```python
from build123d import *

# Parameters (mm, degrees)
F0_W     = 101.6
F0_H     = 50.8
F1_DEPTH = 25.4
F2_W     = 50.8
F2_H     = 25.4
F3_DEPTH = 25.401


with BuildPart() as f1:
    # F0 (on Front) → F1 (new body)
    with BuildSketch(Plane.XZ):
        Rectangle(F0_W, F0_H)
    extrude(amount=F1_DEPTH)

    # F2 (on Front) → F3 (cut, through all)
    with BuildSketch(Plane.XZ):
        with Locations((25.4, 0)):
            Rectangle(F2_W, F2_H)
    extrude(amount=F3_DEPTH, mode=Mode.SUBTRACT)


solid = f1.part
```
The listing builds one solid part. Answer for the finished solid, in the listing's coordinates (mm). A direction names the side the tool comes from. Round coordinates to 2 decimals unless told otherwise and drop trailing zeros. Loops run counter-clockwise (first coordinate to the right, second up) from the corner with the lowest first, then second, coordinate; pieces in that order, holes last. Notation, with made-up numbers: (61, 50) - (85, 50) arc R22 ccw to (85, 61) - close; hole circle Ø7 at (-21, 64). An arc over 180 degrees is marked (long way). Use one line per item in the form item = value. Start each with the question number.
1. Given pin 1 Ø3 at (y, z) = (-5, -10) entering from +X, flat-ended and moving along its own axis, determine where the tip first touches the part or whether it passes through.
2. Consider line 1 (Z direction, x = 1.5, y = -4.25); line 2 (X direction, y = -12.75, z = -4.5). Determine where each line is inside the solid, lowest interval first. Write a range as [from, to].
3. The part is cut by section C-C on z = 9. Determine the outline of the cut face in (x, y), then the cut area to 3 significant figures.
4. The part is cut by section B-B on y = -8.5. Determine the outline of the cut face in (x, z).
5. The part is cut by section A-A on x = 38.5. Determine the outline of the cut face in (y, z).
6. A tool of negligible diameter and unlimited length cuts with its end or side. For faces 1 (the face through (25, -13, -12.7)), 2 (the face through (-12, -25.4, 0)), from which of +Z, -Z, +X, -X, +Y, -Y can it reach the whole face along a straight path? Write none if from no direction.
7. For a pull along Z with two mould halves and no side action, classify faces 3 (the face through (-1, -13, -25.4)), 4 (the face through (0, -13, 0)), 5 (the face through (-1, -13, 25.4)), 6 (the face through (50.8, -13, -19)) as pulls with the +Z half, pulls with the -Z half, needs draft (parallel to the pull), parting line crosses it, or undercut.
Geometry check:
q1.pin_1 = 0
q2.line_1 = [-25.4, -12.7], [12.7, 25.4]
q2.line_2 = [-50.8, 0]
q3.outline = (-50.8, -25.4) - (0, -25.4) - (0, 0) - (-50.8, 0) - close
q3.area = 1,290 mm^2
q4.outline = (-50.8, -25.4) - (50.8, -25.4) - (50.8, -12.7) - (0, -12.7) - (0, 12.7) - (50.8, 12.7) - (50.8, 25.4) - (-50.8, 25.4) - close
q5.outline = (-25.4, -25.4) - (0, -25.4) - (0, -12.7) - (-25.4, -12.7) - close; (-25.4, 12.7) - (0, 12.7) - (0, 25.4) - (-25.4, 25.4) - close
q6.face_1 = +X, +Y, -Y
q6.face_2 = +Z, -Z, +X, -X, -Y
q7.face_3 = pulls with the -Z half
q7.face_4 = undercut
q7.face_5 = pulls with the +Z half
q7.face_6 = needs draft
